```python
from build123d import *

# Parameters (mm, degrees)
F0_W     = 16
F0_H     = 5
F1_DEPTH = 22.5
F3_DEPTH = 9.6


with BuildPart() as f1:
    # F0 (on Front) → F1 (new body)
    with BuildSketch(Plane.XZ):
        with Locations((0, 12.8)):
            Rectangle(F0_W, F0_H)
    extrude(amount=F1_DEPTH)

    # F2 (on face) → F3 (join)
    with BuildSketch(Plane.XY.offset(15.3)):
        with BuildLine():
            Line((-1, -9.25), (-1, -9.813859))
            ThreePointArc((-1, -9.813859), (0, -13), (1, -9.813859))
            Line((1, -9.813859), (1, -9.25))
            Line((1, -9.25), (-1, -9.25))
        make_face()
    extrude(amount=F3_DEPTH)


solid = f1.part
```
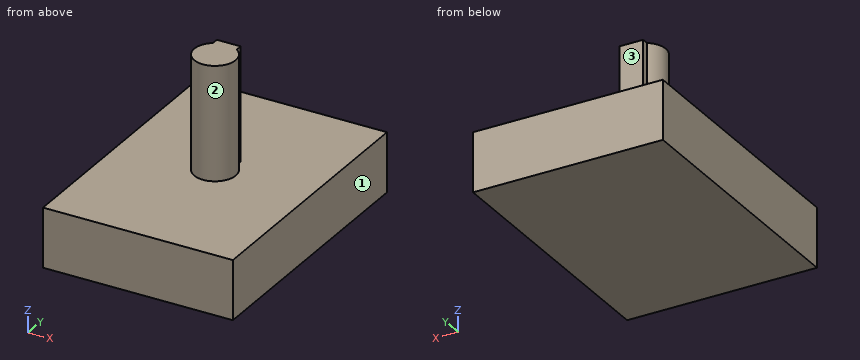
Model file for the job. Use its own axes, mm. Face numbers are marked on the shaded views. A direction names the side the tool comes from. Give positions to 0.01 mm unless a question says otherwise; leave off trailing zeros. Write each loop counter-clockwise with the first axis right and the second up, starting at its lowest first coordinate (ties: lowest second). Pieces come first, ordered by that corner, then holes. Notation, with made-up numbers: (55, 21) - (110, 21) arc R23 cw to (110, 48) - close; hole circle Ø2 at (23.5, -39). An arc over 180 degrees is marked (long way). One line per question, with ' | ' between items. Start each with the question number.
(1) Slice it at D-D on y = -8.75. Write the cut outline in (x, z), plus the area to 3 significant figures.
(2) Slice it at A-A on x = 0. Write the cut outline in (y, z).
(3) Slice it at B-B on y = -11.25. Write the cut outline in (x, z), plus the area to 3 significant figures.
(4) Wall check: line 1 along Z through (x, y) = (3.25, -19); line 2 along Y through (x, z) = (-0.25, 15.5); line 3 along X through (y, z) = (-11.5, 19.5). Give the ranges that are in metal, low to high. Write a range as from..to.
(5) 3-axis set-ups, long thin cutter, end or side, ignore diameter. For the marked faces 1, 2 and 3: which of +Z, -Z, +X, -X, +Y, -Y reach the whole face in a straight line?
(6) Pin check, flat tips, straight feed: P1, Ø5, axis at x = -6.5, y = -9, coming from the +Z side; P2, Ø0.5, axis at y = -9.5, z = 18.5, coming from the -X side; P3, Ø0.5, axis at y = -9.5, z = 19.5, coming from the +X side. Stop position of each tip, or through.
(7) Slice it at C-C on z = 23.5. Write the cut outline in (x, y), plus the area to 3 significant figures.
Results below:
1) outline: (-8, 10.3) - (8, 10.3) - (8, 15.3) - (-8, 15.3) - close | area: 80.0 mm^2
2) outline: (-22.5, 10.3) - (0, 10.3) - (0, 15.3) - (-9.25, 15.3) - (-9.25, 24.9) - (-13, 24.9) - (-13, 15.3) - (-22.5, 15.3) - close
3) outline: (-8, 10.3) - (8, 10.3) - (8, 15.3) - (1.75, 15.3) - (1.75, 24.9) - (-1.75, 24.9) - (-1.75, 15.3) - (-8, 15.3) - close | area: 114 mm^2
4) line 1: 10.3..15.3 | line 2: -12.98..-9.25 | line 3: -1.73..1.73
5) face 1: +Z, -Z, +X, +Y, -Y | face 2: +Z | face 3: +Z, +X, -X, +Y
6) P1: z = 15.3 | P2: x = -1 | P3: x = 1
7) outline: (-1, -9.81) arc R1.75 ccw (long way) to (1, -9.81) - (1, -9.25) - (-1, -9.25) - close | area: 10.3 mm^2
